Verification items for the finished model (mm, model axes). A direction names the side the tool comes from. Give positions to 0.01 mm unless a question says otherwise; leave off trailing zeros. Loops run counter-clockwise (first coordinate to the right, second up) from the corner with the lowest first, then second, coordinate; pieces in that order, holes last. Notation, with made-up numbers: M 68.5,7.5 L 102.5,7.5 A29 ccw 102.5,32.5 Z; hole C 40.25,-10 d10. An arc over 180 degrees is marked long. Use a Markdown table: item, result.
Solid Edge part; units mm, degrees
sketch "Sketch1" plane through (0, 0, 0) normal (1, 0, 0) x (0, 1, 0)
  circle A0 centre (0, 0) radius 12.5
extrude "Extrusionsausprägung_15" add sketch "Sketch1" along normal mid plane 22
sketch "Sketch2" plane through (-11, 0, 0) normal (-1, 0, 0) x (0, -1, 0)
  circle A0 centre (0, 0) radius 15.5
extrude "Extrusionsausprägung_16" add sketch "Sketch2" along normal blind 3
chamfer "Fase_13" distance 2.9 distance2 2.4 1 edges at (-11, 15.5, 0) measured on face at (-11, 10.0233, 10.6433)
sketch "Sketch3" plane through (-14, 0, 0) normal (-1, 0, 0) x (0, 0, -1)
  circle A0 centre (0, 0) radius 8.1
extrude "Extrusionsausschnitt_23" cut sketch "Sketch3" against normal blind 5.2
chamfer "Fase_10" distance 0.75 angle 45 1 edges at (-14, 0, 8.1)
chamfer "Fase_11" distance 0.5 angle 45 1 edges at (-14, 15.5, 0)
mirror "Mirror1" about plane through (0, 0, 0) normal (1, 0, 0) of "Extrusionsausprägung_16", "Extrusionsausschnitt_23", "Fase_10", "Fase_11", "Fase_13"
sketch "Sketch4" plane through (8.8, 0, 0) normal (1, 0, 0) x (0, 0, 1)
  circle A0 centre (0, 0) radius 5.15
extrude "Extrusionsausschnitt_24" cut sketch "Sketch4" against normal blind 20
chamfer "Fase_12" distance 3 angle 45 2 edges at (8.8, 0, -5.15) (-8.8, -5.15, 0)
(1) Gauge pin test, flat ends, axial feed: P1, Ø10, axis at x = -8.5, z = 10, coming from the +Y side; P2, Ø7.5, axis at y = -3.5, z = 5.5, coming from the +X side; P3, Ø1.5, axis at x = 0.5, z = 10, coming from the -Y side; P4, Ø13, axis at y = 0, z = 0, coming from the -X side. Record the tip position at first contact, or that the pin passes through.
Results below:
| item | result |
|---|---|
| P1 | y = 12.83 |
| P2 | x = 14 |
| P3 | y = -8.41 |
| P4 | x = -7.15 |
(2) Set-up check for faces 1 (the cylindrical face through (-11.032, 7.907, 1.756)), 2 (the flat face through (-14, 6.5, -6.5)), 3 (the cylindrical face through (0.154, 11.923, 3.755)), 4 (the cylindrical face through (11.032, -7.907, 1.756)): record each of +Z, -Z, +X, -X, +Y, -Y from which the full face is reachable in a straight line by a thin tool's end or side.
Results below:
| item | result |
|---|---|
| face 1 | -X |
| face 2 | +Z, -Z, -X, +Y, -Y |
| face 3 | none |
| face 4 | +X |
(3) Cross-section at A-A on x = 3.5. Record the cut outline in (y, z), then the cut area to 3 significant figures.
Results below:
| item | result |
|---|---|
| outline | C 0,0 d25; hole C 0,0 d10.3 |
| area | 408 mm^2 |
(4) Material ranges on line 1 (Z direction, x = -2.5, y = 0); line 2 (Z direction, x = -9.75, y = 0); line 3 (X direction, y = 10, z = 8), recorded low to high.
Results below:
| item | result |
|---|---|
| line 1 | -12.5 to -5.15, 5.15 to 12.5 |
| line 2 | -12.5 to -8.1, 8.1 to 12.5 |
| line 3 | -14 to -11.17, 11.17 to 14 |
(5) Draft check along X on faces 5 (the conical face through (-11.15, 2.77, -12.48)), 6 (the cylindrical face through (0.08, -1.55, 4.91)), 7 (the conical face through (-5.985, 5.289, -0.694)), 8 (the conical face through (11.15, 2.77, 12.48)). Enter one of: +X half, -X half, draft (parallel to the pull), parting line (faces both ways), or undercut.
Results below:
| item | result |
|---|---|
| face 5 | undercut |
| face 6 | draft |
| face 7 | -X half |
| face 8 | undercut |
